Source: CAD feature listing. Evaluate the final solid. Frame: model axes, mm. Give positions to 0.01 mm unless a question says otherwise; leave off trailing zeros. Loops run counter-clockwise (first coordinate to the right, second up) from the corner with the lowest first, then second, coordinate; pieces in that order, holes last. Notation, with made-up numbers: (-36, 42) -> (23, 42) arc R8 cw to (23, 56) -> close; hole circle Ø10 at (7.5, 16). An arc over 180 degrees is marked (long way). Answer as a JSON object with one key per item and string values. Group by question number.
Autodesk Inventor part; units mm, degrees
ref_plane "Work Plane1" through (26.8116, 22.4976, 25) normal (0.766, 0.6428, 0) x (-0.6428, 0.766, 0)
ref_plane "Work Plane2" through (17.5, 30.3109, 25) normal (0.5, 0.866, 0) x (-0.866, 0.5, 0)
ref_plane "Work Plane3" through (-17.5, 30.3109, 25) normal (-0.5, 0.866, 0) x (-0.866, -0.5, 0)
sketch "Sketch1" plane through (0, 0, 0) normal (0, 0, 1) x (1, 0, 0)
  circle A0 centre (0, 0) radius 35
  dimension "d0" = 70
extrude "Extrusion1" add sketch "Sketch1" along normal blind 25
chamfer "Chamfer1" distance 2 angle 45 2 edges at (-35, 0, 25) (-35, 0, 0)
sketch "Sketch2" plane through (0, 0, 25) normal (0, 0, 1) x (1, 0, 0)
  line L0 (0, 0) -> (0, 35) construction
  circle A0 centre (0, 0) radius 35 construction
  line L1 (0, 0) -> (35, 0) construction
  line L2 (0, 0) -> (26.8116, 22.4976) construction
  line L3 (0, 0) -> (35, 0) construction
  line L4 (0, 0) -> (17.5, 30.3109) construction
  line L5 (0, 0) -> (35, 0) construction
  line L6 (0, 0) -> (-26.8116, 22.4976) construction
  line L7 (0, 0) -> (-17.5, 30.3109) construction
  dimension "d6" = 40
  dimension "d7" = 60
  dimension "d48" = 60
ref_plane "Work Plane1" through (26.8116, 22.4976, 25) normal (0.766, 0.6428, 0) x (-0.6428, 0.766, 0)
ref_plane "Work Plane2" through (17.5, 30.3109, 25) normal (0.5, 0.866, 0) x (-0.866, 0.5, 0)
ref_plane "Work Plane3" through (-17.5, 30.3109, 25) normal (-0.5, 0.866, 0) x (-0.866, -0.5, 0)
ref_plane "Work Plane4" through (-26.8116, 22.4976, 25) normal (-0.766, 0.6428, 0) x (-0.6428, -0.766, 0)
sketch "Sketch3" plane through (26.8116, 22.4976, 25) normal (0.766, 0.6428, 0) x (-0.6428, 0.766, 0)
  line L0 (-33, 0) -> (33, 0)
  point P0 (0, -25)
  point P1 (0, -14.5)
  dimension "d8" = 14.5
sketch "Sketch4" plane through (17.5, 30.3109, 25) normal (0.5, 0.866, 0) x (-0.866, 0.5, 0)
  line L0 (-33, 0) -> (33, 0)
  point P0 (0, -25)
  point P1 (0, -14.5)
  dimension "d9" = 14.5
sketch "Sketch5" plane through (-17.5, 30.3109, 25) normal (-0.5, 0.866, 0) x (-0.866, -0.5, 0)
  line L0 (-33, 0) -> (33, 0)
  point P0 (0, -25)
  point P1 (0, -14.5)
  dimension "d10" = 14.5
sketch "Sketch6" plane through (-26.8116, 22.4976, 25) normal (-0.766, 0.6428, 0) x (-0.6428, -0.766, 0)
  line L0 (-33, 0) -> (33, 0)
  point P0 (0, -25)
  point P1 (0, -14.5)
  dimension "d11" = 14.5
hole "Hole1" at (-26.8116, 22.4976, 10.5) direction (0.766, -0.6428, 0) diameter 3 depth 8 tip angle 118
hole "Hole2" at (-17.5, 30.3109, 10.5) direction (0.5, -0.866, 0) diameter 3 depth 8 tip angle 118
hole "Hole3" at (17.5, 30.3109, 10.5) direction (-0.5, -0.866, 0) diameter 3 depth 8 tip angle 118
hole "Hole4" at (26.8116, 22.4976, 10.5) direction (-0.766, -0.6428, 0) diameter 3 depth 8 tip angle 118
thread "Thread1"
thread "Thread2"
thread "Thread3"
thread "Thread4"
properties part number "dummy_disc" material "Aluminum 6061"
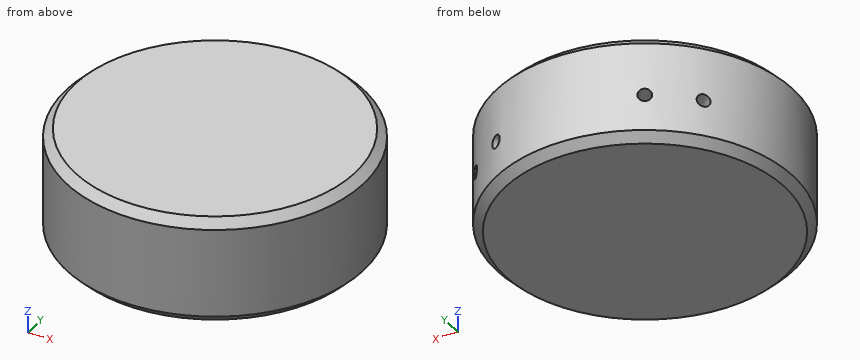
(1) Section query A-A on z = 21.25. Return the cut outline in (x, y).
(2) Material intervals for line 1 (X direction, y = 18.5, z = 10); line 2 (Z direction, x = -16.5, y = 28.5); line 3 (Y direction, x = 24, z = 11), sorted ascending. Write a range as from..to.
(3) First-contact query: pin 1 (12 mm diameter, centred on y = 8, z = 10, fed in from -X); pin 2 (2 mm diameter, centred on x = 18, z = 15, fed in from -Y); pin 3 (10 mm diameter, centred on y = -15.5, z = 6, fed in from -X). Flat tips, straight axial feed; report the tip coordinate or a pass-through.
Result:
{
 "1": {"outline": "circle Ø70 at (0, 0)"},
 "2": {"line 1": "-29.71..-24.25, -19.85..19.85, 24.25..29.71", "line 2": "0..9, 12..25", "line 3": "-25.48..18.29, 21.98..25.48"},
 "3": {"pin 1": "x = -34.94", "pin 2": "y = -30.59", "pin 3": "x = -33.39"}
}
